The listing builds one solid part. Answer for the finished solid, in the listing's coordinates (mm). Face numbers are marked on the shaded views. A direction names the side the tool comes from. Give positions to 0.01 mm unless a question says otherwise; leave off trailing zeros. Write each loop counter-clockwise with the first axis right and the second up, starting at its lowest first coordinate (ties: lowest second). Pieces come first, ordered by that corner, then holes.
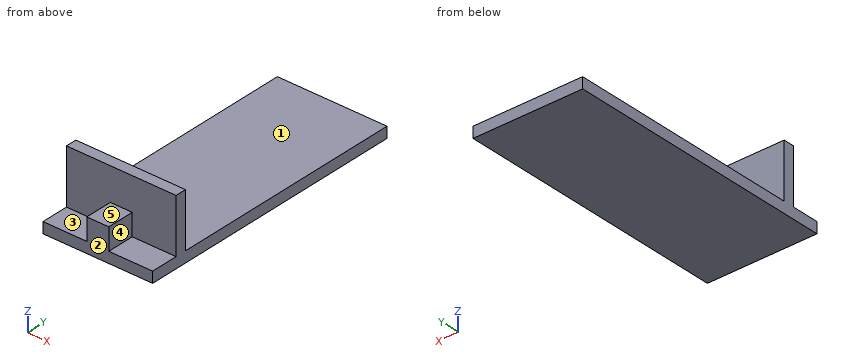
```python
from build123d import *

# Parameters (mm, degrees)
CROQUIS1_W              = 20
CROQUIS1_H              = 2
SALIENTE_EXTRUIR1_DEPTH = 50
CROQUIS2_W              = 4
CROQUIS2_H              = 5
SALIENTE_EXTRUIR2_DEPTH = 4
SALIENTE_EXTRUIR3_DEPTH = 10


with BuildPart() as part:
    # Croquis1 → Saliente-Extruir1 (new body)
    with BuildSketch(Plane(origin=(0, 0, 0), x_dir=(1, 0, 0), z_dir=(0, 1, 0))):
        with Locations((10, 1)):
            Rectangle(CROQUIS1_W, CROQUIS1_H)
    extrude(amount=SALIENTE_EXTRUIR1_DEPTH)

    # Croquis2 → Saliente-Extruir2 (add)
    with BuildSketch(Plane.XY):
        with Locations((10, 2.5)):
            Rectangle(CROQUIS2_W, CROQUIS2_H)
    extrude(amount=SALIENTE_EXTRUIR2_DEPTH)

    # Croquis3 → Saliente-Extruir3 (add)
    with BuildSketch(Plane.XY):
        Polygon((12, 5), (20, 5), (20, 7), (0, 7), (0, 5), align=None)
    extrude(amount=SALIENTE_EXTRUIR3_DEPTH)


solid = part.part
```
Item 1: Which of the six approach directions +Z, -Z, +X, -X, +Y, -Y give full straight-line access (tool end or side, diameter ignored) to the marked faces 1, 2, 3, 4 and 5?
Conclusion:
face 1: +Z, +X, -X, +Y
face 2: +Z, -Z, +X, -X, -Y
face 3: +Z, -X, -Y
face 4: +Z, +X, -Y
face 5: +Z, +X, -X, -Y
Item 2: Consider probe 1 along Z at (x, y) = (1, 28.5); probe 2 along Y at (x, z) = (9, 6.5); probe 3 along X at (y, z) = (2, 0.5). Determine where each line is inside the solid, lowest interval first.
Conclusion:
probe 1: z = -2 to 0
probe 2: y = 5 to 7
probe 3: x = 8 to 12
Item 3: A cutting plane is placed at D-D, the plane y = 15. Give the vertices of the cut face in (x, z), plus the area to 3 significant figures.
Conclusion:
outline: (0, -2) - (20, -2) - (20, 0) - (0, 0) - close
area: 40.0 mm2
Item 4: Each of these flat-tipped pins is pushed along its axis until it touches: P1, Ø6, axis at x = 17, z = 8.5, coming from the +Y side; P2, Ø4, axis at x = 17, y = 1.5, coming from the +Z side; P3, Ø1.2, axis at y = 2.5, z = 3, coming from the -X side; P4, Ø6, axis at x = 10.5, z = 0.5, coming from the -Y side. Where does it stop, or does it pass through?
Conclusion:
P1: stops at y = 7
P2: stops at z = 0
P3: stops at x = 8
P4: stops at y = 0
Item 5: A cutting plane is placed at A-A, the plane x = 4.25. Give the vertices of the cut face in (y, z), plus the area to 3 significant figures.
Conclusion:
outline: (0, -2) - (50, -2) - (50, 0) - (7, 0) - (7, 10) - (5, 10) - (5, 0) - (0, 0) - close
area: 120 mm2
Item 6: A cutting plane is placed at B-B, the plane y = 4. Give the vertices of the cut face in (x, z), plus the area to 3 significant figures.
Conclusion:
outline: (0, -2) - (20, -2) - (20, 0) - (12, 0) - (12, 4) - (8, 4) - (8, 0) - (0, 0) - close
area: 56.0 mm2
Item 7: A cutting plane is placed at C-C, the plane z = 8.25. Give the vertices of the cut face in (x, y), plus the area to 3 significant figures.
Conclusion:
outline: (0, 5) - (20, 5) - (20, 7) - (0, 7) - close
area: 40.0 mm2
